For this review, take the finished solid that the model builds, in its own axes (mm). Face numbers are marked on the shaded views. Round coordinates to 2 decimals unless told otherwise and drop trailing zeros. Loops run counter-clockwise (first coordinate to the right, second up) from the corner with the lowest first, then second, coordinate; pieces in that order, holes last.
1. Consider section A-A on x = -50. State the section outline as (y, z) points, then the cut area to 3 significant figures.
2. Draft analysis for pull direction X (two halves, no side actions). For the marked faces 1 and 2, state which applies: released by +X, released by -X, zero draft, split by the parting line, or undercut.
3. Clearance check with flat-ended pins moving along their axes: pin 1 Ø1.3 at (y, z) = (-0.5, 20.5) entering from -X; pin 2 Ø3 at (x, y) = (-65.5, 1) entering from -Z; pin 3 Ø3 at (y, z) = (1.5, 14) entering from +X. State where each tip first meets the part, or that it passes through.
4. To check wall thickness, follow line 1 along Z through (x, y) = (-3, -1.9); line 2 along X through (y, z) = (-1.45, 13.5); line 3 along Z through (x, y) = (-41.5, 1.4). State the ranges of each line that lie inside material, in increasing order.
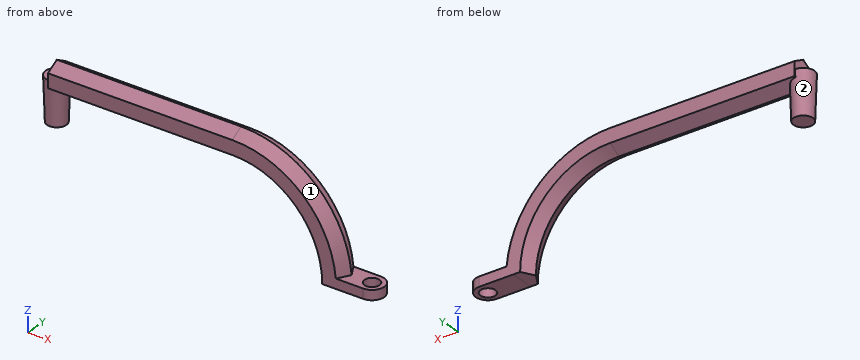
from build123d import *

# Parameters (mm, degrees)
SKETCH_R  = 1.55
PAD_DEPTH = 2


with BuildPart() as part:
    # Sketch → Pad (new body)
    with BuildSketch(Plane.XY):
        with BuildLine():
            Line((0, 2.5), (-7, 2.5))
            Line((-7, 2.5), (-7, -2.5))
            Line((0, -2.5), (-7, -2.5))
            ThreePointArc((0, -2.5), (2.5, 0), (0, 2.5))
        make_face()
        Circle(SKETCH_R, mode=Mode.SUBTRACT)
    extrude(amount=PAD_DEPTH)

    # AdditivePipe: sweep along a path in Sketch001
    with BuildLine(Plane.XZ) as additivepipe_path:
        ThreePointArc((-7, 0), (-12.857864, 14.142136), (-27, 20))
        Line((-27, 20), (-65, 20))
    # Sketch002 → AdditivePipe (sweep)
    with BuildSketch(Plane.XY):
        Polygon((-8.443376, -2.5), (-5.556624, -2.5), (-4.113249, 0), (-5.556624, 2.5), (-8.443376, 2.5), (-9.886751, 0), align=None)
    sweep(path=additivepipe_path.line)

    # Sketch003 (on Face21 of AdditivePipe) → Revolution (revolve)
    with BuildSketch(Plane(origin=(-65, 0, 0), x_dir=(0, -1, 0), z_dir=(-1, 0, 0))):
        Polygon((0, 20), (0, 11), (2, 11), (2.3, 20), align=None)
    revolve(axis=Axis((-65, 0, 0), (0, 0, 1)))


solid = part.part
Resolved:
1. outline: (-2.5, 18.56) - (0, 17.11) - (2.5, 18.56) - (2.5, 21.44) - (0, 22.89) - (-2.5, 21.44) - close
1. area: 21.7 mm2
2. face 1: released by +X
2. face 2: undercut
3. pin 1: stops at x = -67.3
3. pin 2: stops at z = 11
3. pin 3: stops at x = -8.43
4. line 1: z = 0 to 2
4. line 2: x = -66.5 to -63.5, -15.17 to -9.57
4. line 3: z = 17.92 to 22.08
